Read the model definition and answer for the solid it produces. Units are mm, in the model's axes. Face numbers are marked on the shaded views. A direction names the side the tool comes from. Coordinates: 2 decimals unless noted, no trailing zeros. One line per item, written item: value. Start each with the question number.
1. Consider line 1 along Y through (x, z) = (7, 0); line 2 along X through (y, z) = (-5, -5.75); line 3 along X through (y, z) = (7.75, 4.25). Determine where each line is inside the solid, lowest interval first.
2. For the marked faces 1, 2, 3, 4 and 5, determine the directions among +Z, -Z, +X, -X, +Y, -Y from which every point of the face is accessible in a straight line to the end or side of a thin tool.
3. For a pull along Y with two mould halves and no side action, classify the marked faces 6, 7, 8 and 9 as pulls with the +Y half, pulls with the -Y half, needs draft (parallel to the pull), parting line crosses it, or undercut.
4. Given P1, Ø2, axis at x = 3, z = -0.5, coming from the +Y side; P2, Ø3.5, axis at y = 0, z = 0, coming from the +X side; P3, Ø8, axis at x = 7, y = -5.5, coming from the +Z side; P4, Ø1, axis at x = 7, z = 1.5, coming from the -Y side, each flat-ended and moving along its own axis, determine where each tip first touches the part or whether it passes through.
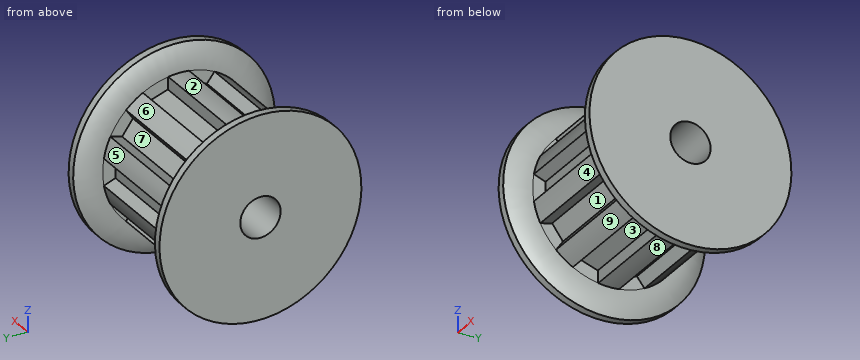
```python
from build123d import *

# Parameters (mm, degrees)
CUT_EXTRUDE1_START = -3
CUT_EXTRUDE1_DEPTH = 12
CIRPATTERN1_COUNT  = 10
SKETCH6_R          = 4
CUT_EXTRUDE2_DEPTH = 6


with BuildPart() as part:
    # Sketch1 → Revolve1 (revolve)
    with BuildSketch(Plane.XY, mode=Mode.PRIVATE) as revolve1_sk:
        with BuildLine():
            Line((-10.5, 2), (10.5, 2))
            Line((10.5, 2), (10.5, 10))
            Line((10.5, 10), (9.75, 10))
            ThreePointArc((9.75, 10), (9.191617437, 8.818070474), (9, 7.525))
            Line((9, 7.525), (-3, 7.525))
            ThreePointArc((-3, 7.525), (-3.191617437, 8.818070474), (-3.75, 10))
            Line((-3.75, 10), (-4.5, 10))
            Line((-4.5, 10), (-4.5, 4))
            Line((-4.5, 4), (-10.5, 4))
            Line((-10.5, 4), (-10.5, 2))
        make_face()
    revolve(revolve1_sk.sketch.rotate(Axis((-10.5, 0, 0), (1, 0, 0)), 90), axis=Axis((-10.5, 0, 0), (1, 0, 0)))

    # Sketch3 → Cut-Extrude1 (cut)
    with BuildSketch(Plane(origin=(0, 0, 0), x_dir=(0, 0, -1), z_dir=(1, 0, 0)).offset(CUT_EXTRUDE1_START)):
        with BuildLine():
            Line((-1.325, 7.407428704), (-0.907223869, 6.259598218))
            Line((-0.907223869, 6.259598218), (0.907223869, 6.259598218))
            Line((0.907223869, 6.259598218), (1.325, 7.407428704))
            ThreePointArc((1.325, 7.407428704), (0, 7.525), (-1.325, 7.407428704))
        make_face()
    cut_extrude1 = extrude(amount=CUT_EXTRUDE1_DEPTH, mode=Mode.SUBTRACT)

    # CirPattern1: Cut-Extrude1 ×10 about axis
    cirpattern1_axis = Axis((0, 0, 0), (1, 0, 0))
    for i in range(1, CIRPATTERN1_COUNT):
        add(cut_extrude1.rotate(cirpattern1_axis, i * 360 / CIRPATTERN1_COUNT), mode=Mode.SUBTRACT)

    # Sketch6 → Cut-Extrude2 (cut)
    with BuildSketch(Plane.ZY.offset(10.5)):
        Circle(SKETCH6_R)
    extrude(amount=-CUT_EXTRUDE2_DEPTH, mode=Mode.SUBTRACT)


solid = part.part
```
Answer block:
1. line 1: y = -6.26 to -2, 2 to 6.26
1. line 2: x = -4.5 to -3, 9 to 10.5
1. line 3: x = -4.5 to -3.2, 9.2 to 10.5
2. face 1: none
2. face 2: +Z
2. face 3: -Z
2. face 4: -Z, -Y
2. face 5: +Z, +Y
3. face 6: pulls with the +Y half
3. face 7: undercut
3. face 8: parting line crosses it
3. face 9: pulls with the -Y half
4. P1: stops at y = 7.41
4. P2: passes through
4. P3: stops at z = 9.66
4. P4: stops at y = -7.41
